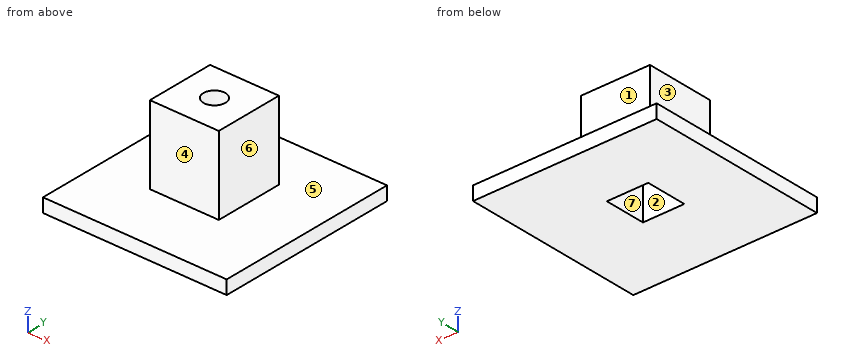
```python
from build123d import *

# Parameters (mm, degrees)
BOX049_W          = 4.5
BOX049_H          = 4.5
BOX049_DEPTH      = 10
BOX048_W          = 20
BOX048_H          = 20
BOX048_DEPTH      = 1.5
CYLINDER034_R     = 1.2
CYLINDER034_DEPTH = 10
BOX047_W          = 4.5
BOX047_H          = 4.5
BOX047_DEPTH      = 10
BOX046_W          = 7.5
BOX046_H          = 7.5
BOX046_DEPTH      = 10


with BuildPart() as cube049:
    # Box049 → Box049 (new body)
    with BuildSketch(Plane(origin=(205.25, 34.25, -5), x_dir=(1, 0, 0), z_dir=(0, 0, 1))):
        with Locations((2.25, 2.25)):
            Rectangle(BOX049_W, BOX049_H)
    extrude(amount=BOX049_DEPTH)


with BuildPart() as cut057:
    # Box048 → Box048 (new body)
    with BuildSketch(Plane(origin=(198, 26, 0), x_dir=(1, 0, 0), z_dir=(0, 0, 1))):
        with Locations((10, 10)):
            Rectangle(BOX048_W, BOX048_H)
    extrude(amount=BOX048_DEPTH)

    # Cut057: cut Cube049
    add(cube049.part, mode=Mode.SUBTRACT)


with BuildPart() as cylinder034:
    # Cylinder034 → Cylinder034 (new body)
    with BuildSketch(Plane(origin=(7.5, 16.5, 105), x_dir=(1, 0, 0), z_dir=(0, 0, 1))):
        Circle(CYLINDER034_R)
    extrude(amount=CYLINDER034_DEPTH)


with BuildPart() as cube047:
    # Box047 → Box047 (new body)
    with BuildSketch(Plane(origin=(5.25, 14.25, 98.5), x_dir=(1, 0, 0), z_dir=(0, 0, 1))):
        with Locations((2.25, 2.25)):
            Rectangle(BOX047_W, BOX047_H)
    extrude(amount=BOX047_DEPTH)


with BuildPart() as testpcbmount:
    # Box046 → Box046 (new body)
    with BuildSketch(Plane(origin=(3.75, 12.75, 100), x_dir=(1, 0, 0), z_dir=(0, 0, 1))):
        with Locations((3.75, 3.75)):
            Rectangle(BOX046_W, BOX046_H)
    extrude(amount=BOX046_DEPTH)

    # Cut055: cut Cube047
    add(cube047.part, mode=Mode.SUBTRACT)

    # Cut056: cut Cylinder034
    add(cylinder034.part, mode=Mode.SUBTRACT)


with BuildPart() as testpcbmount_1:
    # Cut056 placement: moved
    add(testpcbmount.part.moved(Location((200, 20, -100))))

    # Connect006: union Cut057
    add(cut057.part)


solid = testpcbmount_1.part
```
For this review, take the finished solid that the model builds, in its own axes (mm). Face numbers are marked on the shaded views. A direction names the side the tool comes from. Round coordinates to 2 decimals unless told otherwise and drop trailing zeros. Write each loop counter-clockwise with the first axis right and the second up, starting at its lowest first coordinate (ties: lowest second). Pieces come first, ordered by that corner, then holes. Notation, with made-up numbers: (45.25, 7) - (100.25, 7) arc R38 cw to (100.25, 46) - close; hole circle Ø7 at (39.25, 11.5). An arc over 180 degrees is marked (long way). Answer as a JSON object with one key per item and string values.
1. Tool access review of the marked faces 1, 2, 3 and 4: name each direction out of +Z, -Z, +X, -X, +Y, -Y from which nothing blocks a thin tool from reaching the whole face with its end or side.
Response values:
{"face 1": "+Z, +X, -X, +Y", "face 2": "-Z", "face 3": "+Z, -X, +Y, -Y", "face 4": "+Z, +X, -X, -Y"}
2. To check wall thickness, follow line 1 along X through (y, z) = (36.5, 9.6); line 2 along X through (y, z) = (35, 3); line 3 along Y through (x, z) = (207.5, 9). State the ranges of each line that lie inside material, in increasing order.
Response values:
{"line 1": "x = 203.75 to 206.3, 208.7 to 211.25", "line 2": "x = 203.75 to 205.25, 209.75 to 211.25", "line 3": "y = 32.75 to 35.3, 37.7 to 40.25"}
3. We need section C-C on z = 3. Give the boundary of the cut face in (x, y).
Response values:
{"outline": "(203.75, 32.75) - (211.25, 32.75) - (211.25, 40.25) - (203.75, 40.25) - close; hole (205.25, 34.25) - (209.75, 34.25) - (209.75, 38.75) - (205.25, 38.75) - close"}
4. We need section D-D on y = 40. Give the boundary of the cut face in (x, z), then the cut area to 4 significant figures.
Response values:
{"outline": "(198, 0) - (218, 0) - (218, 1.5) - (211.25, 1.5) - (211.25, 10) - (203.75, 10) - (203.75, 1.5) - (198, 1.5) - close", "area": "93.75 mm2"}
5. We need section B-B on x = 207.5. Give the boundary of the cut face in (y, z), then the cut area to 3 significant figures.
Response values:
{"outline": "(26, 0) - (34.25, 0) - (34.25, 8.5) - (35.3, 8.5) - (35.3, 10) - (32.75, 10) - (32.75, 1.5) - (26, 1.5) - close; (37.7, 8.5) - (38.75, 8.5) - (38.75, 0) - (46, 0) - (46, 1.5) - (40.25, 1.5) - (40.25, 10) - (37.7, 10) - close", "area": "51.9 mm2"}
6. We need section A-A on y = 36.5. Give the boundary of the cut face in (x, z).
Response values:
{"outline": "(198, 0) - (205.25, 0) - (205.25, 8.5) - (206.3, 8.5) - (206.3, 10) - (203.75, 10) - (203.75, 1.5) - (198, 1.5) - close; (208.7, 8.5) - (209.75, 8.5) - (209.75, 0) - (218, 0) - (218, 1.5) - (211.25, 1.5) - (211.25, 10) - (208.7, 10) - close"}
7. Draft analysis for pull direction X (two halves, no side actions). For the marked faces 5, 6 and 7, state which applies: +X half, -X half, draft (parallel to the pull), parting line (faces both ways), or undercut.
Response values:
{"face 5": "draft", "face 6": "+X half", "face 7": "undercut"}
8. For pin 1 Ø2 at (x, z) = (205, 8.5) entering from +Y; pin 2 Ø6 at (x, z) = (206, 7.5) entering from -Y; pin 3 Ø2 at (x, y) = (208, 35.5) entering from -Z, all flat-tipped, find the tip position at first contact; note any pin that passes through.
Response values:
{"pin 1": "stops at y = 40.25", "pin 2": "stops at y = 32.75", "pin 3": "stops at z = 8.5"}
